Read the model definition and answer for the solid it produces. Units are mm, in the model's axes. Face numbers are marked on the shaded views. A direction names the side the tool comes from. Round coordinates to 2 decimals unless told otherwise and drop trailing zeros. Write each loop counter-clockwise with the first axis right and the second up, starting at its lowest first coordinate (ties: lowest second). Pieces come first, ordered by that corner, then holes. Notation, with made-up numbers: (-31, 28) -> (2, 28) arc R17 ccw to (2, 46) -> close; hole circle Ø2 at (52, 1.5). An arc over 180 degrees is marked (long way). Return JSON: item names as keys, results as strings. Group by question number.
(1) For the marked faces 5 and 6, determine the directions among +Z, -Z, +X, -X, +Y, -Y from which every point of the face is accessible in a straight line to the end or side of a thin tool.
(2) Given pin 1 (1.4 mm diameter, centred on x = -0.5, z = 4.5, fed in from +Y); pin 2 (0.7 mm diameter, centred on x = 0, y = 84.5, fed in from +Z); pin 3 (2 mm diameter, centred on y = 85.5, z = 1, fed in from +X); pin 4 (2 mm diameter, centred on y = 83.5, z = 5.5, fed in from +X), each flat-ended and moving along its own axis, determine where each tip first touches the part or whether it passes through.
(3) Straight lines are drawn through the part: line 1 (Y direction, x = 2.15, z = 3.75); line 2 (Z direction, x = 1.15, y = 84.8); line 3 (Y direction, x = 2.25, z = 3.5). For each, find the intervals that lie inside material, in ascending order.
(4) The mould has two halves that part along Y. Classify the marked faces 1, 2, 3 and 4: released by +Y, released by -Y, zero draft, split by the parting line, or undercut.
(5) A cutting plane is placed at A-A on z = 3.5. Give the vertices of the cut face in (x, y), then the cut area to 3 significant figures.
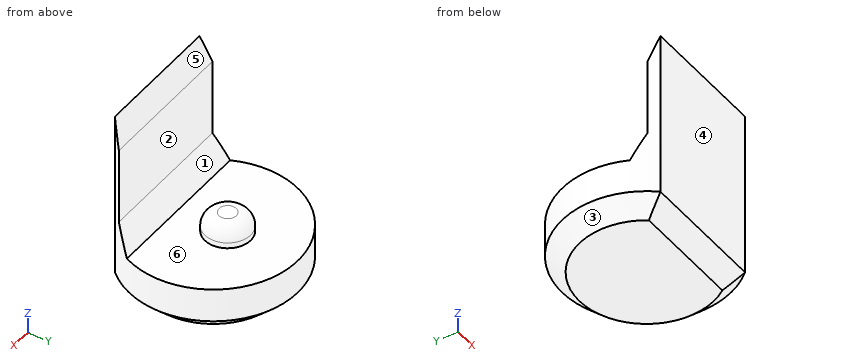
```python
from build123d import *

# Parameters (mm, degrees)
PAD003_DEPTH         = 6.5
POCKET004_DEPTH      = 2.951
POCKET004_DEPTH_BACK = 2.951
SKETCH013_R          = 0.8
PAD006_DEPTH         = 0.7
FILLET_R             = 0.5
CHAMFER004_SIZE      = 0.6


with BuildPart() as part:
    # Sketch004 → Pad003 (new body)
    with BuildSketch(Plane.XY):
        with BuildLine():
            ThreePointArc((2.2, -1.9653244007), (0, 2.95), (-2.2, -1.9653244007))
            Line((-2.2, -1.9653244007), (2.2, -1.9653244007))
        make_face()
    extrude(amount=PAD003_DEPTH)

    # Sketch014 → Pocket004 (cut, two sides)
    with BuildSketch(Plane.YZ) as pocket004_sk:
        Polygon((-1.97, 6.5), (-1.67, 5.5), (-1.67, 2.8), (-1.22, 1.8), (4, 1.8), (4, 6.5), align=None)
    extrude(amount=-POCKET004_DEPTH, mode=Mode.SUBTRACT)
    extrude(pocket004_sk.sketch, amount=POCKET004_DEPTH_BACK, mode=Mode.SUBTRACT)

    # Sketch013 (on Face7 of Pocket004) → Pad006 (join)
    with BuildSketch(Plane.XY.offset(1.8)):
        with Locations((0, 0.5)):
            Circle(SKETCH013_R)
    extrude(amount=PAD006_DEPTH)

    # Fillet
    fillet_edges = [part.edges().sort_by_distance(p)[0] for p in [
        (-0.8, 0.5, 2.5),
    ]]
    fillet(fillet_edges, radius=FILLET_R)

    # Chamfer004
    chamfer004_edges = [part.edges().sort_by_distance(p)[0] for p in [
        (0, 2.95, 0),
        (0, -1.965324, 0),
    ]]
    chamfer(chamfer004_edges, length=CHAMFER004_SIZE)


with BuildPart() as part_1:
    # Body033 placement: moved
    add(part.part.moved(Location((0, 84, 0))))


solid = part_1.part
```
Checks:
{
 "1": {"face 5": "+Z, +X, -X, +Y", "face 6": "+Z"},
 "2": {"pin 1": "stops at y = 82.33", "pin 2": "stops at z = 2.5", "pin 3": "stops at x = 2.91", "pin 4": "passes through"},
 "3": {"line 1": "y = 82.03 to 82.33", "line 2": "z = 0 to 1.8", "line 3": "y = 82.09 to 82.33"},
 "4": {"face 1": "undercut", "face 2": "released by +Y", "face 3": "split by the parting line", "face 4": "released by -Y"},
 "5": {"outline": "(-2.43, 82.33) arc R2.95 ccw to (-2.2, 82.03) -> (2.2, 82.03) arc R2.95 ccw to (2.43, 82.33) -> close", "area": "1.37 mm^2"}
}
